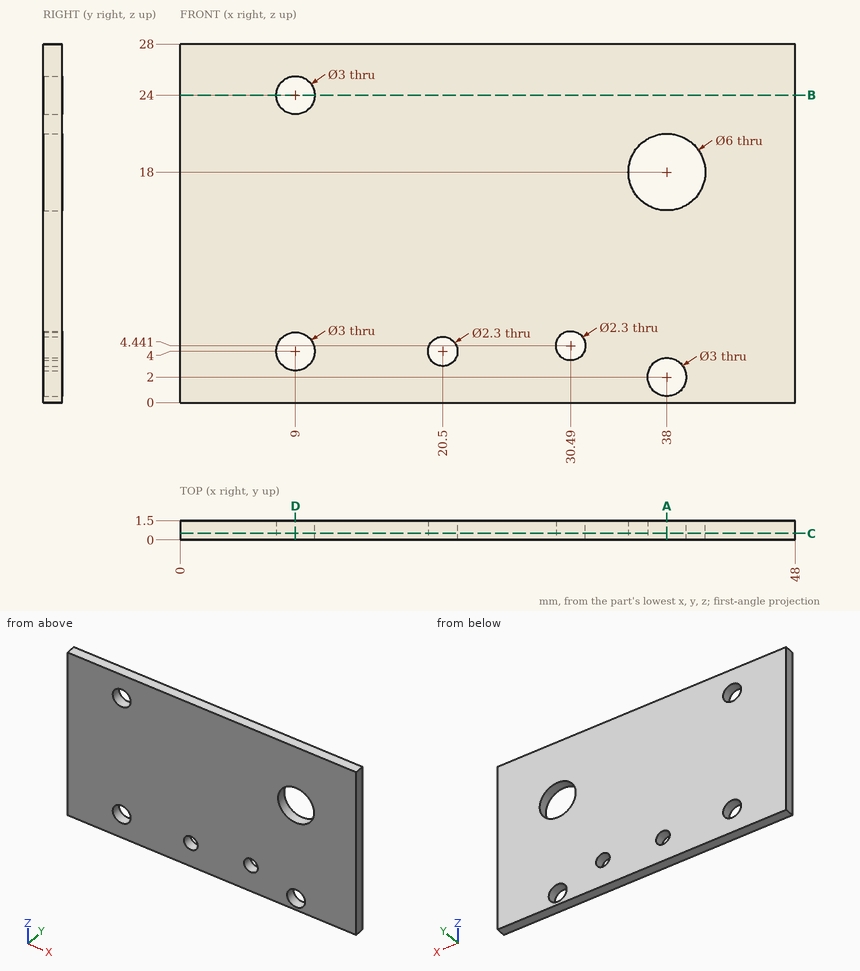
Check sheet for the drawn part. Datum: minimum x, y, z corner. Units: mm. Coordinates: 2 decimals unless noted, no trailing zeros. Loops run counter-clockwise (first coordinate to the right, second up) from the corner with the lowest first, then second, coordinate; pieces in that order, holes last. Notation, with made-up numbers: M 39.25,55 L 72.25,55 A9 cw 72.25,62 Z; hole C 66,9.25 d7. An arc over 180 degrees is marked long. Answer as a JSON object with one key per item and string values.
1. Scan lines: L1, parallel to Z at x = 38, y = 0.4; L2, parallel to Z at x = 9, y = 0.9; L3, parallel to X at y = 1.1, z = 5 (1 decimal). Record each from-to range of solid material in increasing order. Write a range as from..to.
Outcome:
{"L1": "0..0.5, 3.5..15, 21..28", "L2": "0..2.5, 5.5..22.5, 25.5..28", "L3": "0..7.9, 10.1..19.9, 21.1..29.5, 31.5..48"}
2. Sectioned sample at D-D on x = 9. Record the cut outline in (y, z).
Outcome:
{"outline": "M 0,0 L 1.5,0 L 1.5,2.5 L 0,2.5 Z; M 0,5.5 L 1.5,5.5 L 1.5,22.5 L 0,22.5 Z; M 0,25.5 L 1.5,25.5 L 1.5,28 L 0,28 Z"}
3. Sectioned sample at C-C on y = 0.5. Record the cut outline in (x, z), and give its area (3 significant figures).
Outcome:
{"outline": "M 0,0 L 48,0 L 48,28 L 0,28 Z; hole C 9,4 d3; hole C 9,24 d3; hole C 20.5,4 d2.3; hole C 30.49,4.44 d2.3; hole C 38,18 d6; hole C 38,2 d3", "area": "1,290 mm²"}
4. Sectioned sample at A-A on x = 38. Record the cut outline in (y, z).
Outcome:
{"outline": "M 0,0 L 1.5,0 L 1.5,0.5 L 0,0.5 Z; M 0,3.5 L 1.5,3.5 L 1.5,15 L 0,15 Z; M 0,21 L 1.5,21 L 1.5,28 L 0,28 Z"}
5. Sectioned sample at B-B on z = 24. Record the cut outline in (x, y).
Outcome:
{"outline": "M 0,0 L 7.5,0 L 7.5,1.5 L 0,1.5 Z; M 10.5,0 L 48,0 L 48,1.5 L 10.5,1.5 Z"}
